Build history of the part. All positions in model axes, mm. Face numbers are marked on the shaded views. Give positions to 0.01 mm unless a question says otherwise; leave off trailing zeros. Loops run counter-clockwise (first coordinate to the right, second up) from the corner with the lowest first, then second, coordinate; pieces in that order, holes last. Notation, with made-up numbers: (34, 34) -> (67, 34) arc R20 cw to (67, 43) -> close; hole circle Ø11 at (-25.75, -11.75). An arc over 180 degrees is marked (long way). One line per question, with ' | ' between items. Start each with the question number.
(1) Drill centre lines: L1, parallel to X at y = -34, z = 3.4; L2, parallel to Y at x = -37.25, z = 2.9; L3, parallel to Y at x = -38.5, z = 3.85. Where is each one in solid material? Low to high. Write a range as from..to.
(2) Slice it at B-B, the plane z = 0.9. Write the cut outline in (x, y), then the cut area to 3 significant figures.
(3) Mould opens along Y. For the marked faces 1, 2, 3 and 4 say: pulls with the +Y half, pulls with the -Y half, needs draft (parallel to the pull), parting line crosses it, or undercut.
(4) Slice it at A-A, the plane x = -43. Write the cut outline in (y, z).
(5) Slice it at C-C, the plane x = -48. Write the cut outline in (y, z).
```python
from build123d import *

# Parameters (mm, degrees)
SKETCH1_W           = 24
SKETCH1_H           = 80
BOSS_EXTRUDE1_DEPTH = 4
SKETCH2_R           = 4
SKETCH2_R_2         = 1.5
CUT_EXTRUDE1_DEPTH  = 4
FILLET1_R           = 4
SKETCH3_R           = 1.5
CUT_EXTRUDE2_DEPTH  = 4
SKETCH4_W           = 24
SKETCH4_H           = 21.396683756
CUT_EXTRUDE3_DEPTH  = 4


with BuildPart() as part:
    # Sketch1 → Boss-Extrude1 (new body)
    with BuildSketch(Plane.XY):
        with Locations((-45.296675466, -5.049681021)):
            Rectangle(SKETCH1_W, SKETCH1_H)
    extrude(amount=BOSS_EXTRUDE1_DEPTH)

    # Sketch2 → Cut-Extrude1 (cut)
    with BuildSketch(Plane.XY.offset(4)):
        with Locations((-45.296675466, -33.049681021)):
            Circle(SKETCH2_R)
        with Locations((-37.296675466, -33.049681021)):
            Circle(SKETCH2_R_2)
        with Locations((-45.296675466, -41.049681021)):
            Circle(SKETCH2_R_2)
        with Locations((-53.296675466, -33.049681021)):
            Circle(SKETCH2_R_2)
        with Locations((-45.296675466, -25.049681021)):
            Circle(SKETCH2_R_2)
        with Locations((-45.296675466, 30.950318979)):
            Circle(SKETCH2_R_2)
        with Locations((-37.296675466, 22.950318979)):
            Circle(SKETCH2_R_2)
        with Locations((-45.296675466, 14.950318979)):
            Circle(SKETCH2_R_2)
        with Locations((-53.296675466, 22.950318979)):
            Circle(SKETCH2_R_2)
        with Locations((-45.296675466, 22.950318979)):
            Circle(SKETCH2_R)
    extrude(amount=-CUT_EXTRUDE1_DEPTH, mode=Mode.SUBTRACT)

    # Fillet1
    fillet1_edges = [part.edges().sort_by_distance(p)[0] for p in [
        (-57.296675466, 34.950318979, 2),
        (-57.296675466, -45.049681021, 2),
        (-33.296675466, -45.049681021, 2),
        (-33.296675466, 34.950318979, 2),
    ]]
    fillet(fillet1_edges, radius=FILLET1_R)

    # Sketch3 → Cut-Extrude2 (cut)
    with BuildSketch(Plane.XY.offset(4)):
        with Locations((-45.296675466, -5.049681021)):
            Circle(SKETCH3_R)
    extrude(amount=-CUT_EXTRUDE2_DEPTH, mode=Mode.SUBTRACT)

    # Sketch4 → Cut-Extrude3 (cut)
    with BuildSketch(Plane.XY.offset(4)):
        with Locations((-45.296675466, 24.251977101)):
            Rectangle(SKETCH4_W, SKETCH4_H)
    extrude(amount=-CUT_EXTRUDE3_DEPTH, mode=Mode.SUBTRACT)


solid = part.part
```
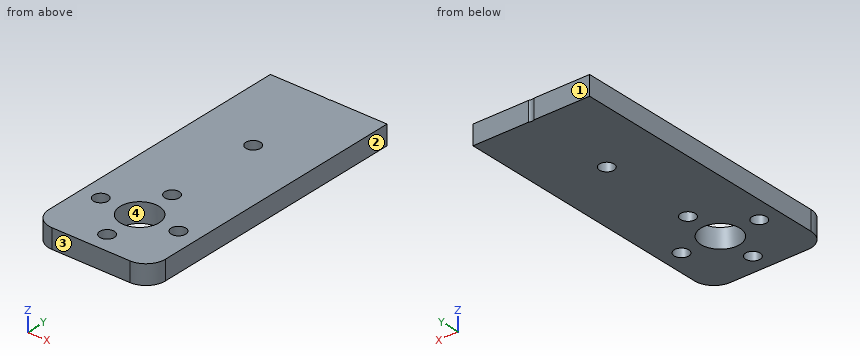
Final values:
1) L1: -57.3..-54.46, -52.14..-49.18, -41.41..-38.46, -36.14..-33.3 | L2: -45.05..-34.55, -31.55..13.55 | L3: -45.05..-33.95, -32.15..13.55
2) outline: (-57.3, -41.05) arc R4 ccw to (-53.3, -45.05) -> (-37.3, -45.05) arc R4 ccw to (-33.3, -41.05) -> (-33.3, 13.55) -> (-44.75, 13.55) arc R1.5 cw to (-45.84, 13.55) -> (-57.3, 13.55) -> close; hole circle Ø3 at (-53.3, -33.05); hole circle Ø8 at (-45.3, -33.05); hole circle Ø3 at (-45.3, -41.05); hole circle Ø3 at (-45.3, -25.05); hole circle Ø3 at (-45.3, -5.05); hole circle Ø3 at (-37.3, -33.05) | area: 1,310 mm2
3) face 1: pulls with the +Y half | face 2: needs draft | face 3: pulls with the -Y half | face 4: undercut
4) outline: (-45.05, 0) -> (-36.32, 0) -> (-36.32, 4) -> (-45.05, 4) -> close; (-29.77, 0) -> (13.55, 0) -> (13.55, 4) -> (-29.77, 4) -> close
5) outline: (-45.05, 0) -> (-36, 0) -> (-36, 4) -> (-45.05, 4) -> close; (-30.1, 0) -> (13.55, 0) -> (13.55, 4) -> (-30.1, 4) -> close
